The figure shows three views and two pictorial views of one solid part (mm, origin at its lowest corner). Answer the questions. Coordinates: 2 decimals unless noted, no trailing zeros. Write each loop counter-clockwise with the first axis right and the second up, starting at its lowest first coordinate (ties: lowest second). Pieces come first, ordered by that corner, then holes.
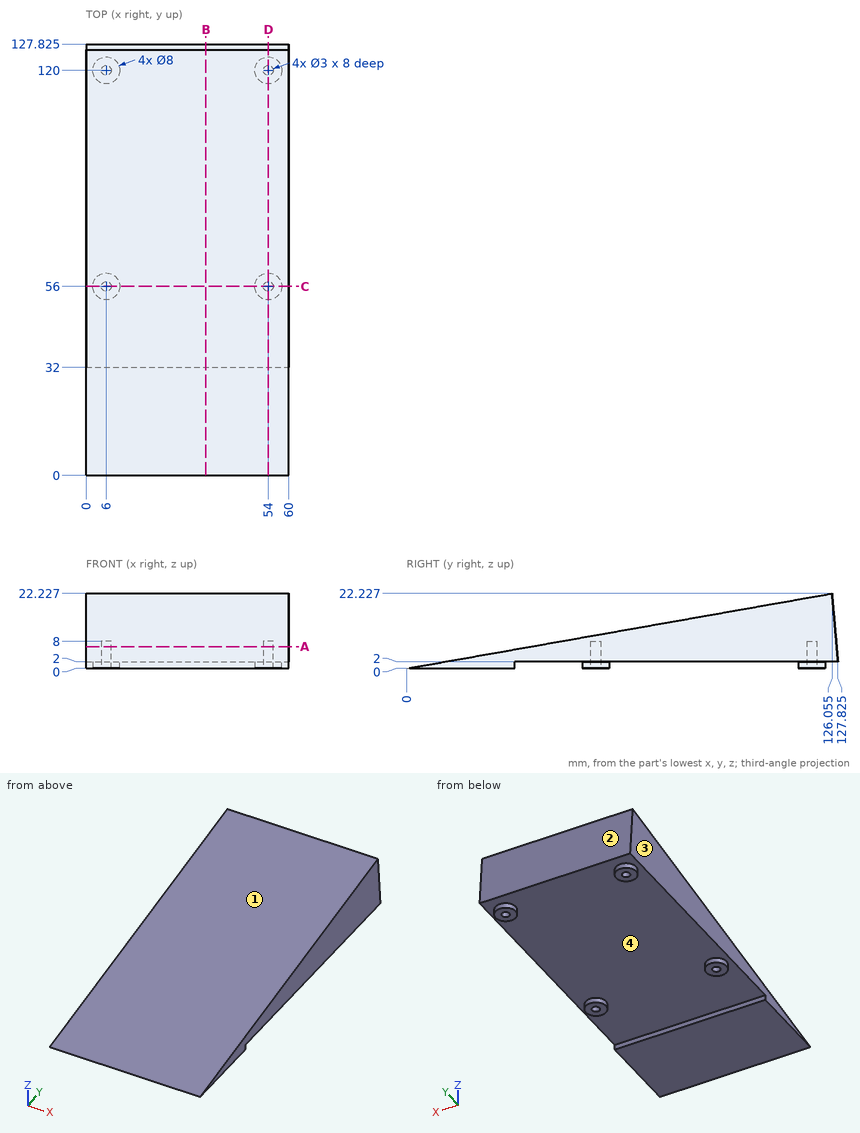
1. Section C-C on y = 56 is taken. Give the vertices of the cut face in (x, z) (1 decimal).
Results found:
outline: (0, 2) - (2, 2) - (2, 0) - (4.5, 0) - (4.5, 8) - (7.5, 8) - (7.5, 0) - (10, 0) - (10, 2) - (50, 2) - (50, 0) - (52.5, 0) - (52.5, 8) - (55.5, 8) - (55.5, 0) - (58, 0) - (58, 2) - (60, 2) - (60, 9.9) - (0, 9.9) - close
2. For a pull along Y with two mould halves and no side action, classify the marked faces 1, 2, 3 and 4 as pulls with the +Y half, pulls with the -Y half, needs draft (parallel to the pull), parting line crosses it, or undercut.
Results found:
face 1: pulls with the -Y half
face 2: pulls with the +Y half
face 3: needs draft
face 4: undercut
3. Section D-D on x = 54 is taken. Give the vertices of the cut face in (y, z) (1 decimal), then the cut area to 3 significant figures.
Results found:
outline: (0, 0) - (32, 0) - (32, 2) - (52, 2) - (52, 0) - (54.5, 0) - (54.5, 8) - (57.5, 8) - (57.5, 0) - (60, 0) - (60, 2) - (116, 2) - (116, 0) - (118.5, 0) - (118.5, 8) - (121.5, 8) - (121.5, 0) - (124, 0) - (124, 2) - (127.8, 2) - (126.1, 22.2) - close
area: 1,210 mm2
4. Flat-ended cylindrical pins translate along their axes: P1, Ø12, axis at x = 14, y = 86.5, coming from the +Z side; P2, Ø1.5, axis at x = 6, y = 120.5, coming from the -Z side; P3, Ø12, axis at x = 41, y = 35.5, coming from the +Z side; P4, Ø3.5, axis at x = 5.5, y = 56.5, coming from the -Z side. Find the tip coordinate at first contact, or state that the pin passes through.
Results found:
P1: stops at z = 16.31
P2: stops at z = 8
P3: stops at z = 7.32
P4: stops at z = 0
5. Section B-B on x = 35.5 is taken. Give the vertices of the cut face in (y, z) (1 decimal).
Results found:
outline: (0, 0) - (32, 0) - (32, 2) - (127.8, 2) - (126.1, 22.2) - close
6. Section A-A on z = 6.5 is taken. Give the vertices of the cut face in (x, y).
Results found:
outline: (0, 36.86) - (60, 36.86) - (60, 127.43) - (0, 127.43) - close; hole circle Ø3 at (6, 56); hole circle Ø3 at (6, 120); hole circle Ø3 at (54, 56); hole circle Ø3 at (54, 120)
7. Find the intervals of material crossed by L1, parallel to X at y = 120, z = 5.5; L2, parallel to X at y = 120, z = 1.75; L3, parallel to Z at x = 24, y = 25.5, in increasing order.
Results found:
L1: x = 0 to 4.5, 7.5 to 52.5, 55.5 to 60
L2: x = 2 to 4.5, 7.5 to 10, 50 to 52.5, 55.5 to 58
L3: z = 0 to 4.5
